Verification items for this drawing (mm, ordinates from the low corner). Coordinates: 2 decimals unless noted, no trailing zeros. Loops run counter-clockwise (first coordinate to the right, second up) from the corner with the lowest first, then second, coordinate; pieces in that order, holes last. Notation, with made-up numbers: (-28, 76) -> (-20, 76) arc R31 cw to (-20, 107) -> close; hole circle Ø11 at (70.25, 84.5). An arc over 180 degrees is marked (long way). Write item = value, one per line.
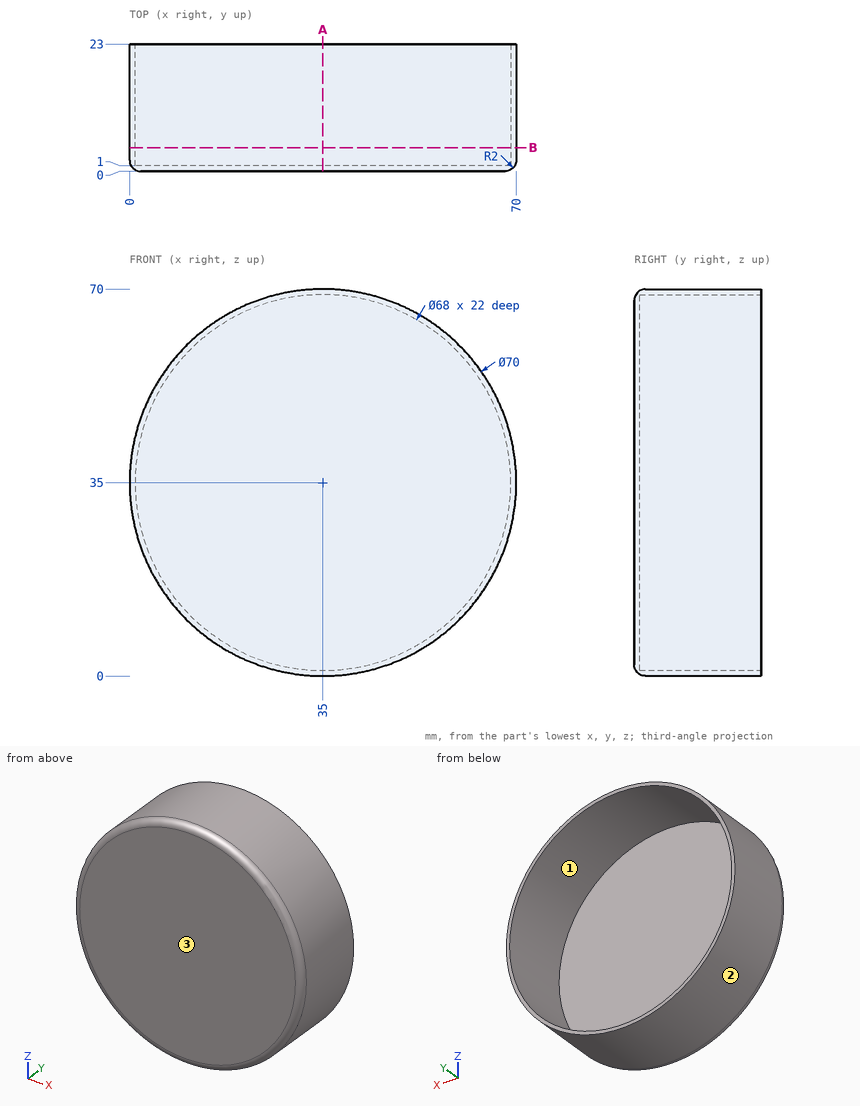
1) Material ranges on line 1 (Z direction, x = 35, y = 15); line 2 (Y direction, x = 40, z = 18.5), recorded low to high.
Ans:
line_1 = 0 to 1, 69 to 70
line_2 = 0 to 1
2) Sectioned sample at A-A, the plane x = 35. Record the cut outline in (y, z).
Ans:
outline = (0, 2) arc R2 ccw to (2, 0) -> (23, 0) -> (23, 1) -> (1, 1) -> (1, 69) -> (23, 69) -> (23, 70) -> (2, 70) arc R2 ccw to (0, 68) -> close
3) Sectioned sample at B-B, the plane y = 4.25. Record the cut outline in (x, z), plus the area to 3 significant figures.
Ans:
outline = circle Ø70 at (35, 35); hole circle Ø68 at (35, 35)
area = 217 mm2
4) Depth check by flat-ended pin: pin 1 Ø3 at (y, z) = (12, 31.5) entering from +X; pin 2 Ø5 at (y, z) = (12, 9) entering from -X; pin 3 Ø1 at (x, y) = (42.5, 19) entering from +Z. Enter the tip coordinate at first touch or a pass-through.
Ans:
pin_1 = 69.94
pin_2 = 9.06
pin_3 = 69.29
5) Release check for a two-part mould opening along Z. For the marked faces 1, 2 and 3 record: pulls with the +Z half, pulls with the -Z half, needs draft (parallel to the pull), parting line crosses it, or undercut.
Ans:
face_1 = undercut
face_2 = parting line crosses it
face_3 = needs draft
